```python
from build123d import *

# Parameters (mm, degrees)
CROQUIS1_W              = 49.8
CROQUIS1_H              = 39.8
CROQUIS1_R              = 2.7
SALIENTE_EXTRUIR1_DEPTH = 6
CORTAR_EXTRUIR1_DEPTH   = 5
CROQUIS3_W              = 4.9
CROQUIS3_H              = 6
CROQUIS3_W_2            = 6
CROQUIS3_H_2            = 6.9
SALIENTE_EXTRUIR2_DEPTH = 7
REDONDEO1_R             = 3
SALIENTE_EXTRUIR3_DEPTH = 3
CROQUIS5_R              = 6.35
CORTAR_EXTRUIR2_DEPTH   = 3
SALIENTE_EXTRUIR4_DEPTH = 10
SALIENTE_EXTRUIR5_DEPTH = 2
CORTAR_EXTRUIR3_START   = -3
CORTAR_EXTRUIR3_DEPTH   = 3


with BuildPart() as part:
    # Croquis1 → Saliente-Extruir1 (new body)
    with BuildSketch(Plane.XY):
        with Locations((-31.963412372, -3.757931034)):
            Rectangle(CROQUIS1_W, CROQUIS1_H)
        with Locations((-52.963412372, 12.342068966)):
            Circle(CROQUIS1_R, mode=Mode.SUBTRACT)
        with Locations((-10.963412372, 12.342068966)):
            Circle(CROQUIS1_R, mode=Mode.SUBTRACT)
        with Locations((-10.963412372, -19.657931034)):
            Circle(CROQUIS1_R, mode=Mode.SUBTRACT)
        with Locations((-52.963412372, -19.657931034)):
            Circle(CROQUIS1_R, mode=Mode.SUBTRACT)
    extrude(amount=SALIENTE_EXTRUIR1_DEPTH)

    # Croquis2 → Cortar-Extruir1 (cut)
    with BuildSketch(Plane.XY.offset(6)):
        with BuildLine():
            Line((-49.963412372, -16.757931034), (-13.963412372, -16.757931034))
            ThreePointArc((-13.963412372, -16.757931034), (-12.54919881, -16.172144597), (-11.963412372, -14.757931034))
            Line((-11.963412372, -14.757931034), (-11.963412372, 7.242068966))
            ThreePointArc((-11.963412372, 7.242068966), (-12.54919881, 8.656282528), (-13.963412372, 9.242068966))
            Line((-13.963412372, 9.242068966), (-49.963412372, 9.242068966))
            ThreePointArc((-49.963412372, 9.242068966), (-51.377625934, 8.656282528), (-51.963412372, 7.242068966))
            Line((-51.963412372, 7.242068966), (-51.963412372, -14.757931034))
            ThreePointArc((-51.963412372, -14.757931034), (-51.377625934, -16.172144597), (-49.963412372, -16.757931034))
        make_face()
    extrude(amount=-CORTAR_EXTRUIR1_DEPTH, mode=Mode.SUBTRACT)

    # Croquis3 → Saliente-Extruir2 (add)
    with BuildSketch(Plane.XY.offset(6)):
        with Locations((-9.513412372, -3.757931034)):
            Rectangle(CROQUIS3_W, CROQUIS3_H)
        with Locations((-31.963412372, -20.207931034)):
            Rectangle(CROQUIS3_W_2, CROQUIS3_H_2)
    extrude(amount=SALIENTE_EXTRUIR2_DEPTH)

    # Redondeo1
    redondeo1_edges = [part.edges().sort_by_distance(p)[0] for p in [
        (-56.863412372, 16.142068966, 3),
        (-7.063412372, 16.142068966, 3),
        (-7.063412372, -23.657931034, 3),
        (-56.863412372, -23.657931034, 3),
    ]]
    fillet(redondeo1_edges, radius=REDONDEO1_R)

    # Croquis4 → Saliente-Extruir3 (add)
    with BuildSketch(Plane(origin=(0, 0, 0), x_dir=(-1, 0, 0), z_dir=(0, 0, -1))):
        with BuildLine():
            Line((56.863412372, 4.242068966), (61.863412372, 4.242068966))
            Line((61.863412372, 4.242068966), (61.863412372, -0.257931034))
            Line((61.863412372, -0.257931034), (57.863412372, -0.257931034))
            ThreePointArc((57.863412372, -0.257931034), (57.358118834, -0.294597605), (56.863412372, -0.403829068))
            Line((56.863412372, -0.403829068), (56.863412372, 4.242068966))
        make_face()
        with BuildLine():
            Line((61.863412372, -11.757931034), (56.863412372, -11.757931034))
            Line((56.863412372, -11.757931034), (56.863412372, -7.112033001))
            ThreePointArc((56.863412372, -7.112033001), (57.358118834, -7.221264464), (57.863412372, -7.257931034))
            Line((57.863412372, -7.257931034), (61.863412372, -7.257931034))
            Line((61.863412372, -7.257931034), (61.863412372, -11.757931034))
        make_face()
    extrude(amount=-SALIENTE_EXTRUIR3_DEPTH)

    # Croquis5 → Cortar-Extruir2 (cut)
    with BuildSketch(Plane.XY.offset(3)):
        with Locations((-57.863412372, -3.757931034)):
            Circle(CROQUIS5_R)
    extrude(amount=CORTAR_EXTRUIR2_DEPTH, mode=Mode.SUBTRACT)

    # Croquis6 → Saliente-Extruir4 (add)
    with BuildSketch(Plane.XY.offset(3)):
        with BuildLine():
            Line((-61.863412372, 4.242068966), (-51.963412372, 4.242068966))
            Line((-51.963412372, 4.242068966), (-48.963412372, 4.242068966))
            Line((-48.963412372, 4.242068966), (-48.963412372, -11.757931034))
            Line((-48.963412372, -11.757931034), (-51.963412372, -11.757931034))
            Line((-51.963412372, -11.757931034), (-61.863412372, -11.757931034))
            Line((-61.863412372, -11.757931034), (-61.863412372, -8.689715701))
            ThreePointArc((-61.863412372, -8.689715701), (-51.513412372, -3.757931034), (-61.863412372, 1.173853632))
            Line((-61.863412372, 1.173853632), (-61.863412372, 4.242068966))
        make_face()
    extrude(amount=SALIENTE_EXTRUIR4_DEPTH)

    # Croquis7 → Saliente-Extruir5 (add)
    with BuildSketch(Plane.XY.offset(1)):
        Polygon((-51.963412372, -3.757931034), (-51.963412372, 4.242068966), (-48.963412372, 4.242068966), (-48.963412372, -11.757931034), (-51.963412372, -11.757931034), align=None)
    extrude(amount=SALIENTE_EXTRUIR5_DEPTH)

    # Croquis8 → Cortar-Extruir3 (cut)
    with BuildSketch(Plane.XY.offset(3).offset(CORTAR_EXTRUIR3_START)):
        with BuildLine():
            Line((-56.863412372, -0.403829068), (-56.863412372, -7.112033001))
            ThreePointArc((-56.863412372, -7.112033001), (-53.509310406, -3.757931034), (-56.863412372, -0.403829068))
        make_face()
    extrude(amount=CORTAR_EXTRUIR3_DEPTH, mode=Mode.SUBTRACT)


solid = part.part
```
Geometry check sheet. Reference: the model listing, model coordinates, mm. A direction names the side the tool comes from. Round coordinates to 2 decimals unless told otherwise and drop trailing zeros. Order: outer loops, then holes, each group sorted by start corner. A loop starts at its lowest first (then second) coordinate and runs counter-clockwise, first axis right, second up. Notation, with made-up numbers: (78, 86.5) -> (100, 86.5) arc R26 cw to (100, 103.5) -> close; hole circle Ø1 at (85.25, 80.5). An arc over 180 degrees is marked (long way). Return JSON: item names as keys, results as strings. Group by question number.
Q1. Section check D-D, the plane y = -3. Record the boundary of the cut face in (x, z).
Q2. Gauge pin test, flat ends, axial feed: pin 1 (13 mm diameter, centred on x = -48.5, y = -20.5, fed in from +Z); pin 2 (5 mm diameter, centred on y = -4.5, z = 8.5, fed in from -X); pin 3 (0.9 mm diameter, centred on x = -59.5, z = 1, fed in from +Y); pin 4 (4 mm diameter, centred on x = -20, z = 9.5, fed in from +Y). Record the tip position at first contact, or that the pin passes through.
Q3. Tool access check on faces 5 (the flat face through (-46, -19, 6)), 6 (the cylindrical face through (-51.362, 8.672, 3.535)), 7 (the flat face through (-18, -17, 6)), 8 (the flat face through (-56.863, 9, 3)), 9 (the flat face through (-60, -7.258, 1)). Record the directions out of +Z, -Z, +X, -X, +Y, -Y that give a thin tool (end or side, any length) a straight path to the whole face; none if there is none.
Q4. Material ranges on probe 1 along X at (y, z) = (4.5, 5.25); probe 2 along X at (y, z) = (10, 5.25); probe 3 along X at (y, z) = (-21, 1), recorded low to high. Write a range as from..to.
Q5. Release check for a two-part mould opening along X. For faces 1 (the flat face through (-32, -16.758, 4)), 2 (the flat face through (-51.963, 6, 4)), 3 (the flat face through (-34.963, -20, 9)), 4 (the flat face through (-7.063, -4, 4)) record: released by +X, released by -X, zero draft, split by the parting line, or undercut.
Q6. Section check A-A, the plane y = 3.5. Record the boundary of the cut face in (x, z).
Q7. Section check B-B, the plane x = -43. Record the boundary of the cut face in (y, z), plus the area to 3 significant figures.
Q8. Section check C-C, the plane z = 7. Record the boundary of the cut face in (x, y), plus the area to 3 significant figures.
Numbers:
{
 "1": {"outline": "(-53.6, 0) -> (-7.06, 0) -> (-7.06, 13) -> (-11.96, 13) -> (-11.96, 1) -> (-48.96, 1) -> (-48.96, 13) -> (-51.56, 13) -> (-51.56, 3) -> (-53.6, 3) -> close"},
 "2": {"pin 1": "z = 6", "pin 2": "x = -52.4", "pin 3": "y = 4.24", "pin 4": "through"},
 "3": {"face 5": "+Z, -X, -Y", "face 6": "+Z", "face 7": "+Z, +X, -Y", "face 8": "+Z, -Z, -X, +Y", "face 9": "+Z, -Z, -X"},
 "4": {"probe 1": "-56.86..-51.96, -11.96..-7.06", "probe 2": "-56.86..-54.31, -51.62..-12.31, -9.62..-7.06", "probe 3": "-56.84..-55.31, -50.62..-13.31, -8.62..-7.08"},
 "5": {"face 1": "undercut", "face 2": "undercut", "face 3": "released by -X", "face 4": "released by +X"},
 "6": {"outline": "(-61.86, 0) -> (-7.06, 0) -> (-7.06, 6) -> (-11.96, 6) -> (-11.96, 1) -> (-48.96, 1) -> (-48.96, 13) -> (-61.86, 13) -> close"},
 "7": {"outline": "(-23.66, 0) -> (16.14, 0) -> (16.14, 6) -> (9.24, 6) -> (9.24, 1) -> (-16.76, 1) -> (-16.76, 6) -> (-23.66, 6) -> close", "area": "109 mm^2"},
 "8": {"outline": "(-61.86, -11.76) -> (-48.96, -11.76) -> (-48.96, 4.24) -> (-61.86, 4.24) -> (-61.86, 1.17) arc R6.35 cw (long way) to (-61.86, -8.69) -> close; (-34.96, -23.66) -> (-28.96, -23.66) -> (-28.96, -16.76) -> (-34.96, -16.76) -> close; (-11.96, -6.76) -> (-7.06, -6.76) -> (-7.06, -0.76) -> (-11.96, -0.76) -> close", "area": "167 mm^2"}
}
